Design review of the part built by this model. Coordinates are the model's own, in mm. A direction names the side the tool comes from. Coordinates: 2 decimals unless noted, no trailing zeros. Write each loop counter-clockwise with the first axis right and the second up, starting at its lowest first coordinate (ties: lowest second). Pieces come first, ordered by that corner, then holes. Notation, with made-up numbers: (-13.5, 32.5) -> (-6.5, 32.5) arc R11 ccw to (-6.5, 37.5) -> close; hole circle Ø10 at (12, -22.5). An arc over 180 degrees is marked (long way). Answer in a Markdown table with one row per item. Add a question column.
Item 1: For faces 4 (the face through (42, -3, -4)), 5 (the face through (4, -3, -4)), 6 (the face through (6, -3, 43)), 7 (the face through (0, -3, 46)), list the 3-axis set-ups (+Z, -Z, +X, -X, +Y, -Y) from which the entire face can be reached by the end or side of a thin tool; tool diameter is ignored.
Item 2: To check wall thickness, follow line 1 (X direction, y = -4, z = 13.5); line 2 (X direction, y = -0.75, z = 45.5); line 3 (X direction, y = -4, z = 50). State the ranges of each line that lie inside material, in increasing order.
Item 3: Take a section at D-D, the plane z = 58. Write out the cut boundary in (x, y).
Item 4: Draft analysis for pull direction Z (two halves, no side actions). For faces 1 (the face through (23, -3, 0)), 2 (the face through (44, -3, -4)), 3 (the face through (8, -3, 43)), state which applies: released by +Z, released by -Z, zero draft, split by the parting line, or undercut.
Item 5: Take a section at A-A, the plane z = 45.5. Write out the cut boundary in (x, y).
Item 6: Take a section at C-C, the plane x = 27. Write out the cut boundary in (y, z), and give its area (3 significant figures).
Item 7: Take a section at B-B, the plane y = -5.25. Write out the cut boundary in (x, z), and give its area (4 significant figures).
Item 8: Clearance check with flat-ended pins moving along their axes: P1, Ø1.9, axis at y = -4.5, z = 11.5, coming from the +X side (3 decimals); P2, Ø3, axis at x = 23.5, y = -4.5, coming from the +Z side; P3, Ø3, axis at y = -2.5, z = -3.5, coming from the -X side. State where each tip first meets the part, or that it passes through.
from build123d import *

# Parameters (mm, degrees)
F0_W     = 2
F0_H     = 7
F1_DEPTH = 6.4


with BuildPart() as f1:
    # F0 (on Front) → F1 (new body)
    with BuildSketch(Plane.XZ):
        Polygon((0, 90), (0, 0), (4, 0), (4, -8), (22, -8), (22, 0), (24, 0), (24, -8), (42, -8), (42, 0), (44, 0), (44, -8), (62, -8), (62, 0), (65, 0), (20, 90), align=None)
        with Locations((7, 13)):
            Rectangle(F0_W, F0_H, mode=Mode.SUBTRACT)
        with Locations((7, 43)):
            Rectangle(F0_W, F0_H, mode=Mode.SUBTRACT)
        with Locations((7, 78)):
            Rectangle(F0_W, F0_H, mode=Mode.SUBTRACT)
    extrude(amount=F1_DEPTH)


solid = f1.part
Answers:
| question | item | result |
|---|---|---|
| 1 | face 4 | -Z, +Y, -Y |
| 1 | face 5 | -Z, -X, +Y, -Y |
| 1 | face 6 | +Y, -Y |
| 1 | face 7 | +Z, -Z, -X, +Y, -Y |
| 2 | line 1 | x = 0 to 6, 8 to 58.25 |
| 2 | line 2 | x = 0 to 6, 8 to 42.25 |
| 2 | line 3 | x = 0 to 40 |
| 3 | outline | (0, -6.4) -> (36, -6.4) -> (36, 0) -> (0, 0) -> close |
| 4 | face 1 | released by -Z |
| 4 | face 2 | zero draft |
| 4 | face 3 | undercut |
| 5 | outline | (0, -6.4) -> (6, -6.4) -> (6, 0) -> (0, 0) -> close; (8, -6.4) -> (42.25, -6.4) -> (42.25, 0) -> (8, 0) -> close |
| 6 | outline | (-6.4, -8) -> (0, -8) -> (0, 76) -> (-6.4, 76) -> close |
| 6 | area | 538 mm^2 |
| 7 | outline | (0, 0) -> (4, 0) -> (4, -8) -> (22, -8) -> (22, 0) -> (24, 0) -> (24, -8) -> (42, -8) -> (42, 0) -> (44, 0) -> (44, -8) -> (62, -8) -> (62, 0) -> (65, 0) -> (20, 90) -> (0, 90) -> close; hole (6, 9.5) -> (8, 9.5) -> (8, 16.5) -> (6, 16.5) -> close; hole (6, 39.5) -> (8, 39.5) -> (8, 46.5) -> (6, 46.5) -> close; hole (6, 74.5) -> (8, 74.5) -> (8, 81.5) -> (6, 81.5) -> close |
| 7 | area | 4,215 mm^2 |
| 8 | P1 | stops at x = 59.725 |
| 8 | P2 | stops at z = 86 |
| 8 | P3 | stops at x = 4 |
